Geometry: see drawing. Coordinates: mm, zero at the bounding-box minimum. Give positions to 0.01 mm unless a question says otherwise; leave off trailing zeros. Write each loop counter-clockwise with the first axis right and the second up, starting at its lowest first coordinate (ties: lowest second). Pieces come first, ordered by that corner, then holes.
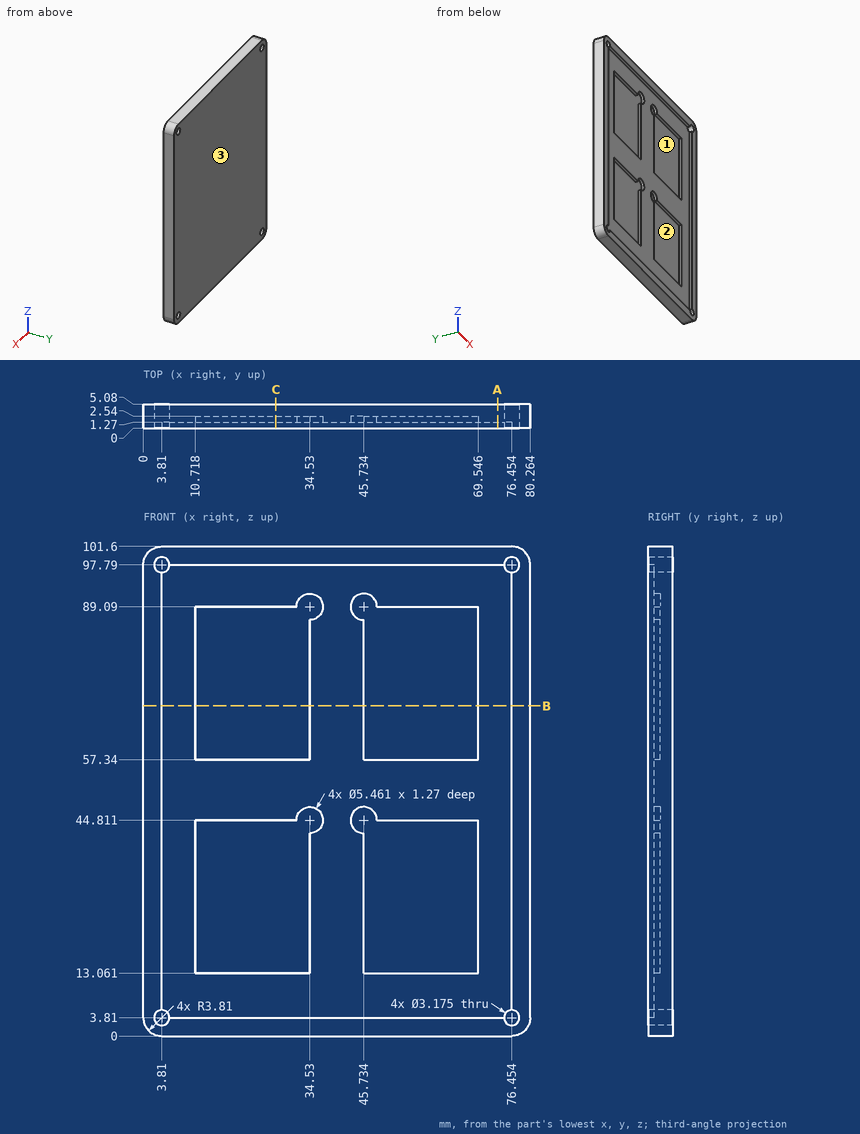
1. Section query C-C (x = 27.5). Return loops of the section in (y, z), plus the area to 3 significant figures.
2. Pin query (flat end, axial travel): P1, Ø4, axis at x = 25.5, z = 61, coming from the -Y side; P2, Ø8, axis at x = 13.5, z = 53, coming from the -Y side; P3, Ø3, axis at x = 76.454, z = 97.79, coming from the -Y side. Return the tip coordinate at first contact, or that it passes through.
3. Section query B-B (z = 68.5). Return loops of the section in (x, y), plus the area to 3 significant figures.
4. Section query A-A (x = 73.5). Return loops of the section in (y, z).
5. Pull-direction query (X, two-part tool) for the marked faces 1, 2 and 3; classes: pulls with the +X half, pulls with the -X half, needs draft (parallel to the pull), parting line crosses it, or undercut.
6. Line query: probe 1 along X at (y, z) = (1.6, 97.79); probe 2 along X at (y, z) = (2.4, 79.5); probe 3 along Z at (x, y) = (14, 1.7). Output: solid intervals per line, ascending.
The answers:
1. outline: (0, 0) - (5.08, 0) - (5.08, 101.6) - (0, 101.6) - (0, 97.79) - (1.27, 97.79) - (1.27, 89.09) - (2.54, 89.09) - (2.54, 57.34) - (1.27, 57.34) - (1.27, 44.81) - (2.54, 44.81) - (2.54, 13.06) - (1.27, 13.06) - (1.27, 3.81) - (0, 3.81) - close
1. area: 316 mm2
2. P1: stops at y = 2.54
2. P2: stops at y = 1.27
2. P3: passes through
3. outline: (0, 0) - (3.81, 0) - (3.81, 1.27) - (10.72, 1.27) - (10.72, 2.54) - (34.53, 2.54) - (34.53, 1.27) - (45.73, 1.27) - (45.73, 2.54) - (69.55, 2.54) - (69.55, 1.27) - (76.45, 1.27) - (76.45, 0) - (80.26, 0) - (80.26, 5.08) - (0, 5.08) - close
3. area: 255 mm2
4. outline: (0, 0) - (5.08, 0) - (5.08, 101.6) - (0, 101.6) - (0, 97.79) - (1.27, 97.79) - (1.27, 3.81) - (0, 3.81) - close
5. face 1: undercut
5. face 2: undercut
5. face 3: needs draft
6. probe 1: x = 0 to 2.22, 5.4 to 74.87, 78.04 to 80.26
6. probe 2: x = 0 to 10.72, 34.53 to 45.73, 69.55 to 80.26
6. probe 3: z = 0 to 13.06, 44.81 to 57.34, 89.09 to 101.6
